Read the model definition and answer for the solid it produces. Units are mm, in the model's axes. Round coordinates to 2 decimals unless told otherwise and drop trailing zeros. Write each loop counter-clockwise with the first axis right and the second up, starting at its lowest first coordinate (ties: lowest second). Pieces come first, ordered by that corner, then holes.
from build123d import *

# Parameters (mm, degrees)
SKETCH1_R           = 5
BOSS_EXTRUDE1_DEPTH = 1.5
SKETCH2_R           = 1.75
CUT_EXTRUDE1_DEPTH  = 8.228416147
CHAMFER1_SIZE       = 1.5
FILLET1_R           = 1


with BuildPart() as part:
    # Sketch1 → Boss-Extrude1 (new body)
    with BuildSketch(Plane.XY):
        Circle(SKETCH1_R)
    extrude(amount=BOSS_EXTRUDE1_DEPTH)

    # Sketch2 → Cut-Extrude1 (cut, through all)
    with BuildSketch(Plane.XY):
        Circle(SKETCH2_R)
    extrude(amount=CUT_EXTRUDE1_DEPTH, mode=Mode.SUBTRACT)

    # Chamfer1
    chamfer1_edges = [part.edges().sort_by_distance(p)[0] for p in [
        (-1.75, 0, 1.5),
    ]]
    chamfer(chamfer1_edges, length=CHAMFER1_SIZE - 0.0001)  # a hair under: the kernel refuses the full size

    # Fillet1
    fillet1_edges = [part.edges().sort_by_distance(p)[0] for p in [
        (-5, 0, 1.5),
    ]]
    fillet(fillet1_edges, radius=FILLET1_R)


solid = part.part
Q1. Section C-C (z = 0.15) is taken. Determine the outline of the cut face in (x, y).
Verdict:
outline: circle Ø10 at (0, 0); hole circle Ø3.8 at (0, 0)
Q2. Flat-ended cylindrical pins translate along their axes: pin 1 Ø5 at (x, y) = (3.5, 2) entering from -Z; pin 2 Ø4 at (x, y) = (0, 0) entering from +Z. Find the tip coordinate at first contact, or state that the pin passes through.
Verdict:
pin 1: stops at z = 0
pin 2: stops at z = 0.25
Q3. Straight lines are drawn through the part: probe 1 along Y at (x, z) = (-0.75, 0.75); probe 2 along X at (y, z) = (-3, 0.1); probe 3 along X at (y, z) = (-0.75, 0.15). For each, find the intervals that lie inside material, in ascending order.
Verdict:
probe 1: y = -4.91 to -2.38, 2.38 to 4.91
probe 2: x = -4 to 4
probe 3: x = -4.94 to -1.75, 1.75 to 4.94
Q4. Section B-B (z = 1.1) is taken. Determine the outline of the cut face in (x, y), then the cut area to 3 significant figures.
Verdict:
outline: circle Ø9.6 at (0, 0); hole circle Ø5.7 at (0, 0)
area: 46.9 mm2
